Work out the finished part from the listing and answer in its coordinate system (mm). A direction names the side the tool comes from. Coordinates: 2 decimals unless noted, no trailing zeros. Loops run counter-clockwise (first coordinate to the right, second up) from the corner with the lowest first, then second, coordinate; pieces in that order, holes last. Notation, with made-up numbers: M -4,43 L 22,43 A24 cw 22,63 Z; hole C 88.25,63.5 d7. An arc over 180 degrees is marked long. Write each question's results on one line, items separated by ' | '.
```python
from build123d import *

# Parameters (mm, degrees)
SKETCH_W     = 25
SKETCH_H     = 8
SKETCH_R     = 1.7
PAD_DEPTH    = 10
SKETCH002_R  = 4
POCKET_DEPTH = 8.001
SKETCH003_W  = 5.75
SKETCH003_H  = 8
SKETCH003_R  = 1.7
PAD001_DEPTH = 6


with BuildPart() as part:
    # Sketch → Pad (new body)
    with BuildSketch(Plane.XY):
        with Locations((9.5, 0)):
            Rectangle(SKETCH_W, SKETCH_H)
        Circle(SKETCH_R, mode=Mode.SUBTRACT)
        with Locations((19, 0)):
            Circle(SKETCH_R, mode=Mode.SUBTRACT)
    extrude(amount=PAD_DEPTH)

    # Sketch002 → Pocket (cut, through all)
    with BuildSketch(Plane.XZ.offset(4)):
        with Locations((9.5, -1)):
            Circle(SKETCH002_R)
    extrude(amount=-POCKET_DEPTH, mode=Mode.SUBTRACT)

    # Sketch003 → Pad001 (new body)
    with BuildSketch(Plane.XY.offset(10)):
        with Locations((-0.125, 0)):
            Rectangle(SKETCH003_W, SKETCH003_H)
        Circle(SKETCH003_R, mode=Mode.SUBTRACT)
        with Locations((19.125, 0)):
            Rectangle(SKETCH003_W, SKETCH003_H)
        with Locations((19, 0)):
            Circle(SKETCH003_R, mode=Mode.SUBTRACT)
    extrude(amount=PAD001_DEPTH)


solid = part.part
```
1) Find section C-C, the plane y = 0. Give the vertices of the cut face in (x, z).
Check result:
outline: M -3,0 L -1.7,0 L -1.7,16 L -3,16 Z; M 1.7,0 L 5.63,0 A4 cw 13.37,0 L 17.3,0 L 17.3,16 L 16.25,16 L 16.25,10 L 2.75,10 L 2.75,16 L 1.7,16 Z; M 20.7,0 L 22,0 L 22,16 L 20.7,16 Z
2) Straight lines are drawn through the part: probe 1 along Y at (x, z) = (0, 3.5); probe 2 along X at (y, z) = (1.25, 13.5); probe 3 along X at (y, z) = (-1.25, 1.5). For each, find the intervals that lie inside material, in ascending order. Write a range as [from, to].
Check result:
probe 1: [-4, -1.7], [1.7, 4] | probe 2: [-3, -1.15], [1.15, 2.75], [16.25, 17.85], [20.15, 22] | probe 3: [-3, -1.15], [1.15, 6.38], [12.62, 17.85], [20.15, 22]
3) Given pin 1 Ø6 at (x, z) = (8, 14.5) entering from +Y, flat-ended and moving along its own axis, determine where the tip first touches the part or whether it passes through.
Check result:
pin 1: through
4) Find section A-A, the plane z = 12.5. Give the vertices of the cut face in (x, y).
Check result:
outline: M -3,-4 L 2.75,-4 L 2.75,4 L -3,4 Z; M 16.25,-4 L 22,-4 L 22,4 L 16.25,4 Z; hole C 0,0 d3.4; hole C 19,0 d3.4
5) For a pull along X with two mould halves and no side action, classify faces 3 (the face through (19, 2, 16)), 4 (the face through (22, 0, 8)), 5 (the face through (9.6, -0.1, 3)) as released by +X, released by -X, zero draft, split by the parting line, or undercut.
Check result:
face 3: zero draft | face 4: released by +X | face 5: undercut
6) Find section B-B, the plane x = 0. Give the vertices of the cut face in (y, z), and give its area (3 significant figures).
Check result:
outline: M -4,0 L -1.7,0 L -1.7,16 L -4,16 Z; M 1.7,0 L 4,0 L 4,16 L 1.7,16 Z | area: 73.6 mm^2
7) Find section D-D, the plane z = 7.5. Give the vertices of the cut face in (x, y), and give its area (3 significant figures).
Check result:
outline: M -3,-4 L 22,-4 L 22,4 L -3,4 Z; hole C 0,0 d3.4; hole C 19,0 d3.4 | area: 182 mm^2
8) Which of the six approach directions +Z, -Z, +X, -X, +Y, -Y give full straight-line access (tool end or side, diameter ignored) to faces 1 (the face through (17, 0, 0)), 2 (the face through (2.75, 0, 13))?
Check result:
face 1: -Z, +X, -X, +Y, -Y | face 2: +Z, +Y, -Y
